```python
from build123d import *

# Parameters (mm, degrees)
F0_W     = 20
F0_H     = 35
F1_DEPTH = 20
F3_R     = 3.175
F4_DEPTH = 10


# Not quite as in the source:
# - a feature names something its author has since deleted; it is built from what else it names


with BuildPart() as f1:
    # F0 (on Front) → F1 (new body)
    with BuildSketch(Plane.XZ):
        with Locations((-160, 52.5)):
            Rectangle(F0_W, F0_H)
        with Locations((-160, -17.5)):
            Rectangle(F0_W, F0_H)
        Polygon((170, -70), (170, 70), (150, 70), (-150, 70), (-150, 35), (-150, 0), (-150, -35), (-150, -70), (150, -70), align=None)
    extrude(amount=-F1_DEPTH)

    # F3 (on face) → F4 (cut)
    with BuildSketch(Plane(origin=(0, 20, 0), x_dir=(-1, 0, 0), z_dir=(0, 1, 0))):
        with Locations((-160.0000113249, 35.0000448525)):
            Circle(F3_R)
        with Locations((-160.0000560284, 0)):
            Circle(F3_R)
        with Locations((-160.0000113249, -35.0000634789)):
            Circle(F3_R)
    extrude(amount=-F4_DEPTH, mode=Mode.SUBTRACT)


solid = f1.part
```
For this review, take the finished solid that the model builds, in its own axes (mm). A direction names the side the tool comes from. Round coordinates to 2 decimals unless told otherwise and drop trailing zeros. Write each loop counter-clockwise with the first axis right and the second up, starting at its lowest first coordinate (ties: lowest second). Pieces come first, ordered by that corner, then holes. Notation, with made-up numbers: (5.5, 10) - (31.5, 10) arc R27 cw to (31.5, 28) - close; hole circle Ø10 at (40, -15.75). An arc over 180 degrees is marked (long way). Put each result on its own line as item: value.
Q1. Insertion check: pin 1 Ø1.9 at (x, z) = (161, 34.5) entering from +Y; pin 2 Ø10 at (x, y) = (-162, 7.5) entering from -Z; pin 3 Ø2 at (y, z) = (4, 31.5) entering from -X. Each pin has a flat end and moves straight along its axis. Give the tip position at first contact, or say it passes through.
Solved:
pin 1: stops at y = 10
pin 2: stops at z = -35
pin 3: stops at x = -150
Q2. Wall thickness on probe 1 along X at (y, z) = (12.5, 36); probe 2 along X at (y, z) = (15.75, 6); probe 3 along X at (y, z) = (14.5, 34): over which ranges is each line inside the solid? List them lowest first.
Solved:
probe 1: x = -170 to 156.99, 163.01 to 170
probe 2: x = -150 to 170
probe 3: x = -150 to 156.99, 163.01 to 170
Q3. We need section A-A (y = 4.25). Give the boundary of the cut face in (x, z).
Solved:
outline: (-170, -35) - (-150, -35) - (-150, -70) - (170, -70) - (170, 70) - (-170, 70) - (-170, 35) - (-150, 35) - (-150, 0) - (-170, 0) - close
Q4. Machinability: for faces 1 (the face through (-160, 10, 0)), 2 (the face through (160.41, 15.07, 38.15)), 3 (the face through (-150, 10, -52)), which of the approach directions +Z, -Z, +X, -X, +Y, -Y give a long, thin tool a straight path to every point of the face, cutting with its end or side? Answer none if there is none.
Solved:
face 1: -X, +Y, -Y
face 2: +Y
face 3: -Z, -X, +Y, -Y
